from build123d import *

# Parameters (mm, degrees)
F0_W     = 1500
F0_H     = 400
F0_W_2   = 1400
F0_H_2   = 300
F1_DEPTH = 50
F2_W     = 50
F2_H     = 50
F3_DEPTH = 100


with BuildPart() as f1:
    # F0 (on Top) → F1 (new body)
    with BuildSketch(Plane.XY):
        with Locations((750, 200)):
            Rectangle(F0_W, F0_H)
        with Locations((750, 200)):
            Rectangle(F0_W_2, F0_H_2, mode=Mode.SUBTRACT)
    extrude(amount=F1_DEPTH)

    # F2 (on face) → F3 (join)
    with BuildSketch(Plane.XY.offset(50)):
        with Locations((25, 375)):
            Rectangle(F2_W, F2_H)
        with Locations((25, 25)):
            Rectangle(F2_W, F2_H)
        with Locations((1475, 375)):
            Rectangle(F2_W, F2_H)
        with Locations((1475, 25)):
            Rectangle(F2_W, F2_H)
    extrude(amount=F3_DEPTH)


solid = f1.part
The listing builds one solid part. Answer for the finished solid, in the listing's coordinates (mm). A direction names the side the tool comes from. Coordinates: 2 decimals unless noted, no trailing zeros. Loops run counter-clockwise (first coordinate to the right, second up) from the corner with the lowest first, then second, coordinate; pieces in that order, holes last.
1) Find section D-D on y = 25. Write down the section's boundary in (x, z), then the cut area to 3 significant figures.
2) Find section C-C on y = 180.5. Write down the section's boundary in (x, z), then the cut area to 3 significant figures.
3) Determine the mould class of faces 1 (the face through (25, 25, 150)), 2 (the face through (746, 400, 36)), 3 (the face through (25, 350, 99)) for opening direction Y: pulls with the +Y half, pulls with the -Y half, needs draft (parallel to the pull), parting line crosses it, or undercut.
4) Find the intervals of material crossed by L1, parallel to Y at x = 1225, z = 35; L2, parallel to X at y = 92.5, z = 16; L3, parallel to Z at x = 279.5, y = 357.5, in increasing order.
5) Find section A-A on z = 95. Write down the section's boundary in (x, y), then the cut area to 3 significant figures.
6) Flat-ended cylindrical pins translate along their axes: pin 1 Ø3 at (y, z) = (170.5, 40) entering from -X; pin 2 Ø15 at (x, y) = (561.5, 381.5) entering from +Z. Find the tip coordinate at first contact, or state that the pin passes through.
7) A tool of negligible diameter and unlimited length cuts with its end or side. For faces 4 (the face through (50, 375, 99)), 5 (the face through (1475, 202, 50)), 6 (the face through (1450, 198, 25)), from which of +Z, -Z, +X, -X, +Y, -Y can it reach the whole face along a straight path? Write none if from no direction.
8) Find section B-B on x = 1197. Write down the section's boundary in (y, z), then the cut area to 3 significant figures.
Values:
1. outline: (0, 0) - (1500, 0) - (1500, 150) - (1450, 150) - (1450, 50) - (50, 50) - (50, 150) - (0, 150) - close
1. area: 85,000 mm2
2. outline: (0, 0) - (50, 0) - (50, 50) - (0, 50) - close; (1450, 0) - (1500, 0) - (1500, 50) - (1450, 50) - close
2. area: 5,000 mm2
3. face 1: needs draft
3. face 2: pulls with the +Y half
3. face 3: undercut
4. L1: y = 0 to 50, 350 to 400
4. L2: x = 0 to 50, 1450 to 1500
4. L3: z = 0 to 50
5. outline: (0, 0) - (50, 0) - (50, 50) - (0, 50) - close; (0, 350) - (50, 350) - (50, 400) - (0, 400) - close; (1450, 0) - (1500, 0) - (1500, 50) - (1450, 50) - close; (1450, 350) - (1500, 350) - (1500, 400) - (1450, 400) - close
5. area: 10,000 mm2
6. pin 1: stops at x = 0
6. pin 2: stops at z = 50
7. face 4: +Z, +Y, -Y
7. face 5: +Z, +X, -X
7. face 6: +Z, -Z
8. outline: (0, 0) - (50, 0) - (50, 50) - (0, 50) - close; (350, 0) - (400, 0) - (400, 50) - (350, 50) - close
8. area: 5,000 mm2
